Source: three-view drawing plus pictorial views. Frame: mm from the lowest corner of the part. A direction names the side the tool comes from. Give positions to 0.01 mm unless a question says otherwise; leave off trailing zeros. Order: outer loops, then holes, each group sorted by start corner. A loop starts at its lowest first (then second) coordinate and runs counter-clockwise, first axis right, second up. Notation, with made-up numbers: (-15.75, 45) -> (42.25, 45) arc R29 ccw to (42.25, 66) -> close; hole circle Ø7 at (-28, -8.5). An arc over 180 degrees is marked (long way). One line per question, with ' | ' between items.
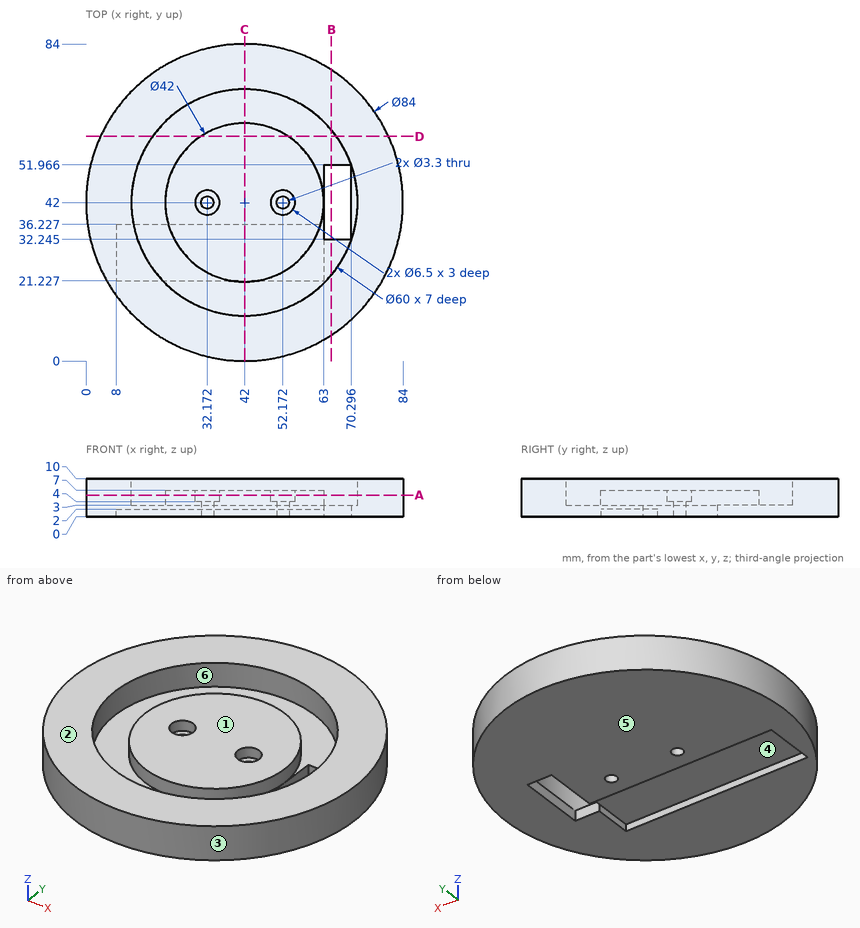
1) Section D-D on y = 59.5. Return loops of the section in (x, z).
Check result:
outline: (3.82, 0) -> (80.18, 0) -> (80.18, 10) -> (66.37, 10) -> (66.37, 3) -> (53.61, 3) -> (53.61, 7) -> (30.39, 7) -> (30.39, 3) -> (17.63, 3) -> (17.63, 10) -> (3.82, 10) -> close
2) Material intervals for probe 1 along X at (y, z) = (42, 8.75); probe 2 along X at (y, z) = (25.5, 5) (1 decimal); probe 3 along X at (y, z) = (56.5, 4.5) (1 decimal), sorted ascending. Write a range as from..to.
Check result:
probe 1: x = 0..12, 72..84 | probe 2: x = 3.4..16.9, 29..55, 67.1..80.6 | probe 3: x = 2.6..15.7, 26.8..57.2, 68.3..81.4
3) Pull-direction query (X, two-part tool) for the marked faces 1, 2 and 3; classes: +X half, -X half, draft (parallel to the pull), parting line (faces both ways), or undercut.
Check result:
face 1: undercut | face 2: draft | face 3: parting line
4) Section A-A on z = 5.75. Return loops of the section in (x, y).
Check result:
outline: circle Ø84 at (42, 42); circle Ø42 at (42, 42); hole circle Ø60 at (42, 42); hole circle Ø6.5 at (32.17, 42); hole circle Ø6.5 at (52.17, 42)
5) Contact query for flat-ended pins moving along their axis: pin 1 Ø1.6 at (y, z) = (29.5, 1) entering from +X; pin 2 Ø2 at (x, z) = (28.5, 1.5) entering from -Y; pin 3 Ø1.5 at (x, z) = (32.5, 3) entering from +Y. Output: stop coordinate, or through.
Check result:
pin 1: stops at x = 82.34 | pin 2: stops at y = 1.9 | pin 3: stops at y = 83.08
6) Set-up query: the marked faces 4, 5 and 6. Return all of +Z, -Z, +X, -X, +Y, -Y with unobstructed straight access to the full face (end or side cutting, diameter ignored); none if empty.
Check result:
face 4: -Z | face 5: -Z, +X, -X, +Y, -Y | face 6: +Z
7) Section B-B on x = 65. Return loops of the section in (y, z) (1 decimal), plus the area to 3 significant figures.
Check result:
outline: (6.9, 0) -> (32.2, 0) -> (32.2, 3) -> (22.7, 3) -> (22.7, 10) -> (6.9, 10) -> close; (52, 0) -> (77.1, 0) -> (77.1, 10) -> (61.3, 10) -> (61.3, 3) -> (52, 3) -> close | area: 374 mm^2
8) Section C-C on x = 42. Return loops of the section in (y, z).
Check result:
outline: (0, 0) -> (21.23, 0) -> (21.23, 2) -> (36.23, 2) -> (36.23, 0) -> (84, 0) -> (84, 10) -> (72, 10) -> (72, 3) -> (63, 3) -> (63, 7) -> (21, 7) -> (21, 3) -> (12, 3) -> (12, 10) -> (0, 10) -> close
